```python
from build123d import *

# Parameters (mm, degrees)
F1_DEPTH       = 25
F2_W           = 7
F2_H           = 19
F3_DEPTH       = 37.501
F5_D           = 4.2
F5_DEPTH       = 12
F5_TIP         = 1.2618073
F7_D           = 6.4
F7_CBORE_D     = 11
F7_CBORE_DEPTH = 7
F9_R           = 6
F10_DEPTH      = 20


with BuildPart() as f1:
    # F0 (on Front) → F1 (new body, symmetric)
    with BuildSketch(Plane.XZ):
        Polygon((-17.5, 0), (0, 0), (0, 24), (-37.5, 24), (-37.5, -11), (-27.5, -11), (-27.5, -1), (-17.5, -1), align=None)
    extrude(amount=F1_DEPTH, both=True)

    # F2 (on Right) → F3 (cut, through all)
    with BuildSketch(Plane.YZ):
        with Locations((21.5, 14.5)):
            Rectangle(F2_W, F2_H)
    extrude(amount=-F3_DEPTH, mode=Mode.SUBTRACT)

    # F5
    with Locations(Plane(origin=(0, 0, -11), x_dir=(1, 0, 0), z_dir=(0, 0, -1))):
        with Locations((-32.5, 18), (-32.5, -18)):
            Hole(F5_D / 2, depth=F5_DEPTH)
            with Locations((0, 0, -(F5_DEPTH + F5_TIP / 2))):  # 118° drill point
                Cone(0, F5_D / 2, F5_TIP, mode=Mode.SUBTRACT)

    # F7 (through all)
    with Locations(Plane.XZ.offset(25)):
        with Locations((-27.5, 15)):
            CounterBoreHole(F7_D / 2, F7_CBORE_D / 2, F7_CBORE_DEPTH)

    # F8: F1 across plane


with BuildPart() as f1_1:
    add(f1.part)
    add(f1.part.mirror(Plane.YZ))

    # F9 (on face) → F10 (cut)
    with BuildSketch(Plane.XZ.offset(25)):
        with Locations((0, 13)):
            Circle(F9_R)
    extrude(amount=-F10_DEPTH, mode=Mode.SUBTRACT)


solid = f1_1.part
```
Model file for the job. Use its own axes, mm. A direction names the side the tool comes from. Coordinates: 2 decimals unless noted, no trailing zeros. Order: outer loops, then holes, each group sorted by start corner. A loop starts at its lowest first (then second) coordinate and runs counter-clockwise, first axis right, second up. Notation, with made-up numbers: (39, 8.25) - (61, 8.25) arc R15 ccw to (61, 30.25) - close; hole circle Ø3 at (-25.5, -2.75). An arc over 180 degrees is marked (long way). Return JSON: item names as keys, results as strings. Group by question number.
1) Saw through at D-D, the plane x = 0. Write the cut outline in (y, z).
2) Saw through at C-C, the plane z = 15. Write the cut outline in (x, y).
3) Saw through at A-A, the plane z = -3. Write the cut outline in (x, y).
4) Mould opens along Z. For faces 6 (the cylindrical face through (31.9, -21.5, 11.7)), 7 (the flat face through (37.5, 0, 7)), 8 (the cylindrical face through (-1.301, -15.14, 7.143)), 9 (the flat face through (-1, 21, 5)) say: released by +Z, released by -Z, zero draft, split by the parting line, or undercut.
5) Flat gauge pins, fed straight in: P1, Ø1, axis at x = -6, y = 7.5, coming from the -Z side; P2, Ø11, axis at x = -20, y = 9.5, coming from the -Z side; P3, Ø3.5, axis at x = 29, z = 15.5, coming from the -Y side. Where does each tip first touch, or does it go through?
6) Tool access for faces 1 (the flat face through (23, 0, -1)), 2 (the flat face through (-1, 18, 14)), 3 (the flat face through (0, -5, 13)), 4 (the flat face through (-1, -4, 24)), 5 (the cylindrical face through (30.952, -19.419, -4.916)): list every direction of +Z, -Z, +X, -X, +Y, -Y with a clear straight run to the whole face (end or side of a thin tool).
7) Probe line 1 (Y direction, x = -32.5, z = -4.75); line 2 (X direction, y = -4, z = -6.5); line 3 (X direction, y = -18, z = -3.5). List the from-to ranges inside material, lowest first. Write a range as from..to.
8) Saw through at B-B, the plane y = 13.5. Write the cut outline in (x, z), plus the area to 3 significant figures.
Values found:
{
 "1": {"outline": "(-25, 0) - (25, 0) - (25, 5) - (18, 5) - (18, 24) - (-25, 24) - (-25, 19) - (-5, 19) - (-5, 7) - (-25, 7) - close"},
 "2": {"outline": "(-37.5, -25) - (-33, -25) - (-33, -18) - (-30.7, -18) - (-30.7, 18) - (-37.5, 18) - close; (-24.3, -18) - (-22, -18) - (-22, -25) - (-5.66, -25) - (-5.66, -5) - (5.66, -5) - (5.66, -25) - (22, -25) - (22, -18) - (24.3, -18) - (24.3, 18) - (-24.3, 18) - close; (30.7, -18) - (33, -18) - (33, -25) - (37.5, -25) - (37.5, 18) - (30.7, 18) - close"},
 "3": {"outline": "(-37.5, -25) - (-27.5, -25) - (-27.5, 25) - (-37.5, 25) - close; (27.5, -25) - (37.5, -25) - (37.5, 25) - (27.5, 25) - close; hole circle Ø4.2 at (-32.5, -18); hole circle Ø4.2 at (-32.5, 18); hole circle Ø4.2 at (32.5, -18); hole circle Ø4.2 at (32.5, 18)"},
 "4": {"face 6": "undercut", "face 7": "zero draft", "face 8": "undercut", "face 9": "released by +Z"},
 "5": {"P1": "stops at z = 0", "P2": "stops at z = -1", "P3": "stops at y = -18"},
 "6": {"face 1": "-Z, +Y, -Y", "face 2": "+Z, +X, -X, +Y", "face 3": "-Y", "face 4": "+Z, +X, -X, +Y, -Y", "face 5": "-Z"},
 "7": {"line 1": "y = -25..-20.1, -15.9..15.9, 20.1..25", "line 2": "x = -37.5..-27.5, 27.5..37.5", "line 3": "x = -37.5..-34.6, -30.4..-27.5, 27.5..30.4, 34.6..37.5"},
 "8": {"outline": "(-37.5, -11) - (-27.5, -11) - (-27.5, -1) - (-17.5, -1) - (-17.5, 0) - (17.5, 0) - (17.5, -1) - (27.5, -1) - (27.5, -11) - (37.5, -11) - (37.5, 24) - (-37.5, 24) - close; hole circle Ø6.4 at (-27.5, 15); hole circle Ø6.4 at (27.5, 15)", "area": "1,980 mm²"}
}
